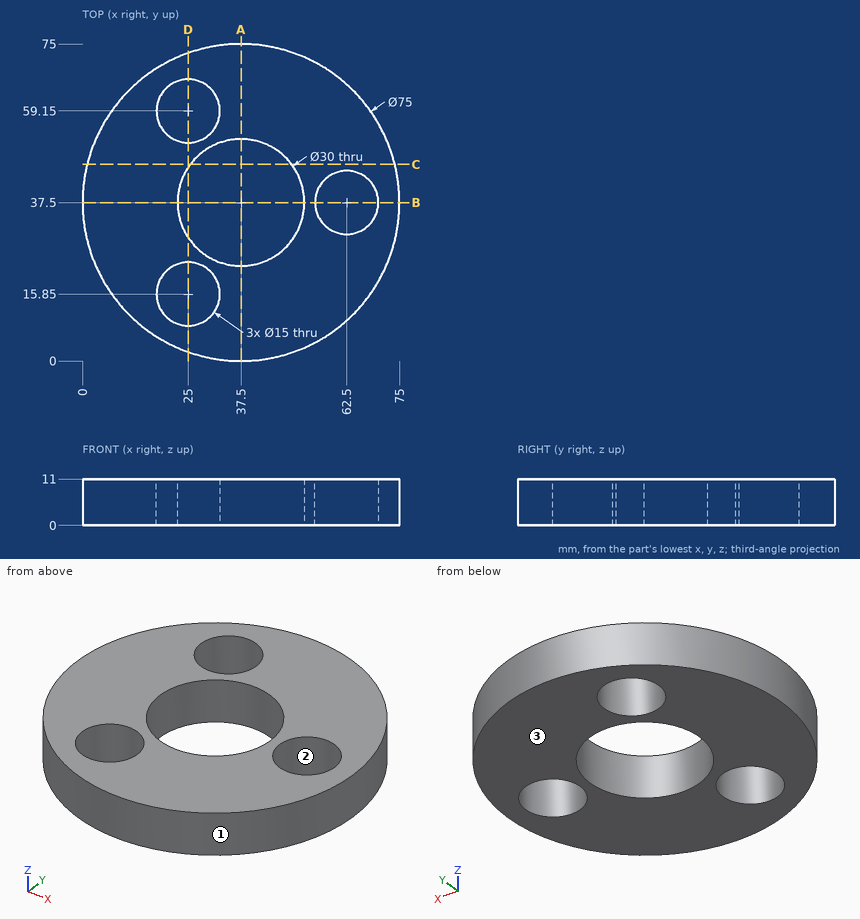
For this review, use the dimensioned drawing (mm, ordinates from the lowest corner) and the shaded views. Give positions to 0.01 mm unless a question says otherwise; leave off trailing zeros. Order: outer loops, then holes, each group sorted by start corner. A loop starts at its lowest first (then second) coordinate and runs counter-clockwise, first axis right, second up. Notation, with made-up numbers: (-34.5, 77) - (-19.5, 77) arc R18 cw to (-19.5, 106) - close; hole circle Ø6 at (46, 73.25). An arc over 180 degrees is marked (long way). Write item = value, one per line. Start each with the question number.
Q1. We need section D-D on x = 25. State the section outline as (y, z) points.
Q2. We need section C-C on y = 46.5. State the section outline as (x, z) points.
Q3. To check wall thickness, follow L1, parallel to X at y = 42, z = 9; L2, parallel to Y at x = 25, z = 5; L3, parallel to X at y = 39, z = 9.75. State the ranges of each line that lie inside material, in increasing order. Write a range as from..to.
Q4. Mouldability with a two-part tool opening along Y and no side actions: class the marked faces 1, 2 and 3 as released by +Y, released by -Y, zero draft, split by the parting line, or undercut.
Q5. We need section A-A on x = 37.5. State the section outline as (y, z) points, plus the area to 3 significant figures.
Q6. We need section B-B on y = 37.5. State the section outline as (x, z) points, plus the area to 3 significant figures.
Q7. Clearance check with flat-ended pins moving along their axes: pin 1 Ø3 at (y, z) = (60, 7) entering from +X; pin 2 Ø5 at (x, z) = (47, 9) entering from +Y; pin 3 Ø5 at (y, z) = (21, 2) entering from +X. State where each tip first meets the part, or that it passes through.
Working result:
q1.outline = (2.14, 0) - (8.35, 0) - (8.35, 11) - (2.14, 11) - close; (23.35, 0) - (29.21, 0) - (29.21, 11) - (23.35, 11) - close; (45.79, 0) - (51.65, 0) - (51.65, 11) - (45.79, 11) - close; (66.65, 0) - (72.86, 0) - (72.86, 11) - (66.65, 11) - close
q2.outline = (1.1, 0) - (25.5, 0) - (25.5, 11) - (1.1, 11) - close; (49.5, 0) - (73.9, 0) - (73.9, 11) - (49.5, 11) - close
q3.L1 = 0.27..23.19, 51.81..56.5, 68.5..74.73
q3.L2 = 2.14..8.35, 23.35..29.21, 45.79..51.65, 66.65..72.86
q3.L3 = 0.03..22.58, 52.42..55.15, 69.85..74.97
q4.face_1 = split by the parting line
q4.face_2 = undercut
q4.face_3 = zero draft
q5.outline = (0, 0) - (22.5, 0) - (22.5, 11) - (0, 11) - close; (52.5, 0) - (75, 0) - (75, 11) - (52.5, 11) - close
q5.area = 495 mm²
q6.outline = (0, 0) - (22.5, 0) - (22.5, 11) - (0, 11) - close; (52.5, 0) - (55, 0) - (55, 11) - (52.5, 11) - close; (70, 0) - (75, 0) - (75, 11) - (70, 11) - close
q6.area = 330 mm²
q7.pin_1 = 68.57
q7.pin_2 = 74.34
q7.pin_3 = 72.29
